```python
from build123d import *

# Parameters (mm, degrees)
CROQUIS1_R              = 7.5
SALIENTE_EXTRUIR1_DEPTH = 7.5
SALIENTE_EXTRUIR2_START = 15
SALIENTE_EXTRUIR2_DEPTH = 15
CROQUIS3_R              = 2.1
CORTAR_EXTRUIR2_DEPTH   = 19.371173071


with BuildPart() as part:
    # Croquis1 → Saliente-Extruir1 (new, symmetric)
    with BuildSketch(Plane(origin=(0, 0, 0), x_dir=(1, 0, 0), z_dir=(0, 1, 0))):
        with Locations(Location((0, 0, 0), (0, 0, 270))):
            Circle(CROQUIS1_R)
    extrude(amount=SALIENTE_EXTRUIR1_DEPTH, both=True)

    # Croquis2 → Saliente-Extruir2 (add)
    with BuildSketch(Plane(origin=(0, 7.5, 0), x_dir=(1, 0, 0), z_dir=(0, 1, 0)).offset(SALIENTE_EXTRUIR2_START)):
        with BuildLine():
            Line((2.1, -7.2), (-7.5, 0))
            ThreePointArc((-7.5, 0), (-4.5, -6), (2.1, -7.2))
        make_face()
    extrude(amount=-SALIENTE_EXTRUIR2_DEPTH)

    # Croquis3 → Cortar-Extruir2 (cut, through all)
    with BuildSketch(Plane(origin=(0, 7.5, 0), x_dir=(1, 0, 0), z_dir=(0, 1, 0))):
        with Locations(Location((0, 0, 0), (0, 0, 270))):
            Circle(CROQUIS3_R)
    extrude(amount=-CORTAR_EXTRUIR2_DEPTH, mode=Mode.SUBTRACT)


solid = part.part
```
Read the model definition and answer for the solid it produces. Units are mm, in the model's axes. A direction names the side the tool comes from. Round coordinates to 2 decimals unless told otherwise and drop trailing zeros. Write each loop counter-clockwise with the first axis right and the second up, starting at its lowest first coordinate (ties: lowest second). Pieces come first, ordered by that corner, then holes. Notation, with made-up numbers: (80, 82.25) -> (99, 82.25) arc R29 cw to (99, 113.25) -> close; hole circle Ø11 at (12, -7.5). An arc over 180 degrees is marked (long way). Answer in a Markdown table with one row per item. Add a question column.
1) Find section C-C, the plane z = 6. Determine the outline of the cut face in (x, y), and give its area (3 significant figures).
2) Which of the six approach directions +Z, -Z, +X, -X, +Y, -Y give full straight-line access (tool end or side, diameter ignored) to faces 4 (the face through (-4, 22.5, 5)), 5 (the face through (2, 7.5, -2))?
3) Consider line 1 (X direction, y = 4.5, z = 0); line 2 (Y direction, x = -2.25, z = 0.5); line 3 (Z direction, x = -1.5, y = 15.75). Determine where each line is inside the solid, lowest interval first.
4) Find section D-D, the plane y = 0. Determine the outline of the cut face in (x, z), and give its area (3 significant figures).
5) Find section A-A, the plane z = -1.5. Determine the outline of the cut face in (x, y).
6) Determine the mould class of faces 1 (the face through (0.631, 0.105, 2.003)), 2 (the face through (-2, -7.5, 2)), 3 (the face through (-3.54, 7.71, 6.61)) for opening direction X: pulls with the +X half, pulls with the -X half, needs draft (parallel to the pull), parting line crosses it, or undercut.
7) Find section B-B, the plane x = 1.75. Determine the outline of the cut face in (y, z).
8) Given P1, Ø1, axis at x = 5.5, y = -2, coming from the -Z side; P2, Ø8, axis at x = -4.5, y = 3.5, coming from the -Z side; P3, Ø8, axis at x = -1, z = -3, coming from the +Y side, each flat-ended and moving along its own axis, determine where each tip first touches the part or whether it passes through.
Findings below:
| question | item | result |
|---|---|---|
| 1 | outline | (-4.5, -7.5) -> (4.5, -7.5) -> (4.5, 7.5) -> (0.5, 7.5) -> (0.5, 22.5) -> (-4.5, 22.5) -> close |
| 1 | area | 210 mm² |
| 2 | face 4 | +Z, -Z, +X, -X, +Y |
| 2 | face 5 | -Z, +X, +Y |
| 3 | line 1 | -7.5 to -2.1, 2.1 to 7.5 |
| 3 | line 2 | -7.5 to 7.5 |
| 3 | line 3 | 4.5 to 7.35 |
| 4 | outline | circle Ø15 at (0, 0); hole circle Ø4.2 at (0, 0) |
| 4 | area | 163 mm² |
| 5 | outline | (-7.35, -7.5) -> (-1.47, -7.5) -> (-1.47, 7.5) -> (-7.35, 7.5) -> close; (1.47, -7.5) -> (7.35, -7.5) -> (7.35, 7.5) -> (1.47, 7.5) -> close |
| 6 | face 1 | undercut |
| 6 | face 2 | needs draft |
| 6 | face 3 | parting line crosses it |
| 7 | outline | (-7.5, -7.29) -> (7.5, -7.29) -> (7.5, -1.16) -> (-7.5, -1.16) -> close; (-7.5, 1.16) -> (7.5, 1.16) -> (7.5, 6.94) -> (22.5, 6.94) -> (22.5, 7.29) -> (-7.5, 7.29) -> close |
| 8 | P1 | z = -5.59 |
| 8 | P2 | z = -7.48 |
| 8 | P3 | y = 7.5 |
